Can you work these out from the model? Positions are in its coordinate system, mm. Face numbers are marked on the shaded views. Coordinates: 2 decimals unless noted, no trailing zeros. Loops run counter-clockwise (first coordinate to the right, second up) from the corner with the lowest first, then second, coordinate; pieces in that order, holes last. Notation, with made-up numbers: M 45,1.5 L 57,1.5 A18 cw 57,29.5 Z; hole C 83,-6 d7. An arc over 180 degrees is marked long. Answer as a JSON object with one key per item and string values. Group by question number.
Item 1: Suppose I cut it at A-A (x = 480). Write out the boundary of the cut face in (y, z).
Item 2: Suppose I cut it at D-D (y = -1327.5). Write out the boundary of the cut face in (x, z).
Item 3: Suppose I cut it at C-C (x = 410.5). Write out the boundary of the cut face in (y, z), then the cut area to 3 significant figures.
Item 4: Suppose I cut it at B-B (y = -1341.5). Write out the boundary of the cut face in (x, z), then the cut area to 3 significant figures.
Item 5: We'd pull the mould along X, two halves only. Please class the marked faces 1, 2, 3 and 4: +X half, -X half, draft (parallel to the pull), parting line (faces both ways), or undercut.
Item 6: If I drill on line 1 (X direction, y = -1322, z = 14.25); line 2 (X direction, y = -1331.5, z = 1.5); line 3 (Z direction, x = 560, y = -1330.5), over which ranges is the centre line in solid material (lowest first)?
Item 7: I'm going to push flat-ended pins straight in: pin 1 Ø3 at (x, y) = (397.81, -1294.47) entering from +Z; pin 2 Ø2.5 at (x, z) = (500.5, 2) entering from +Y; pin 3 Ø1.2 at (x, z) = (473, 16) entering from -Y. Where does each tip first touch, or does it pass through?
```python
from build123d import *

# Parameters (mm, degrees)
SKETCH1_W               = 214
SKETCH1_H               = 75.8
BOSS_EXTRUDE1_DEPTH     = 17
BOSSEXTENTION_DEPTH     = 214
SHELLIT_T               = -3
SKETCH7_W               = 208
SKETCH7_H               = 4
CUT_EXTRUDE4_DEPTH      = 3
SKETCH3_R               = 1.375
MOUNTING_HOLES_DEPTH    = 1479.493115905
PI_HOLE_DEPTH           = 8
CHAMFER1_START          = 8
CHAMFER1_DEPTH          = 2
CHAMFER1_START_2        = -970
CHAMFER1_2_DEPTH        = 1.564999152
FILLET1_R               = 2
SKETCH11_R              = 1.7
CUT_EXTRUDE5_DEPTH      = 893.868694268
CUT_EXTRUDE6_DEPTH      = 893.868694268
CUT_EXTRUDE6_DEPTH_BACK = 1
SKETCH12_R              = 2.75


with BuildPart() as part:
    # Sketch1 → Boss-Extrude1 (new body)
    with BuildSketch(Plane.XY):
        with Locations((466.705697041, -1324.673912477)):
            Rectangle(SKETCH1_W, SKETCH1_H)
    extrude(amount=BOSS_EXTRUDE1_DEPTH)

    # Sketch6 → BossExtention (add)
    with BuildSketch(Plane(origin=(573.705697041, 0, 0), x_dir=(0, 0, -1), z_dir=(1, 0, 0))):
        Polygon((-17, -1286.773912477), (-12.75, -1279.412696544), (0, -1286.773912477), align=None)
    extrude(amount=-BOSSEXTENTION_DEPTH)

    # Shellit
    shellit_openings = [part.faces().sort_by_distance(p)[0] for p in [
        (466.705697041, -1324.673912477, 17),
    ]]
    offset(amount=SHELLIT_T, openings=shellit_openings, kind=Kind.INTERSECTION)

    # Sketch7 → Cut-Extrude4 (cut)
    with BuildSketch(Plane.XY.offset(17)):
        with Locations((466.705697041, -1290.773912477)):
            Rectangle(SKETCH7_W, SKETCH7_H)
    extrude(amount=-CUT_EXTRUDE4_DEPTH, mode=Mode.SUBTRACT)

    # Sketch3 → Mounting Holes (cut, through all)
    with BuildSketch(Plane.XY.offset(3)):
        with Locations((397.805697041, -1294.473912477)):
            Circle(SKETCH3_R)
        with Locations((511.805697041, -1294.473912477)):
            Circle(SKETCH3_R)
        with Locations((397.805697041, -1353.573912477)):
            Circle(SKETCH3_R)
        with Locations((511.805697041, -1353.573912477)):
            Circle(SKETCH3_R)
    extrude(amount=-MOUNTING_HOLES_DEPTH, mode=Mode.SUBTRACT)

    # Sketch4 → PI_Hole (cut)
    with BuildSketch(Plane(origin=(0, 0, 0), x_dir=(-1, 0, 0), z_dir=(0, 0, -1))):
        with BuildLine():
            Line((-404.705697041, -1355.573912477), (-454.805697041, -1355.573912477))
            ThreePointArc((-454.805697041, -1355.573912477), (-456.219910604, -1356.159698914), (-456.805697041, -1357.573912477))
            Line((-456.805697041, -1357.573912477), (-456.805697041, -1358.073912477))
            ThreePointArc((-456.805697041, -1358.073912477), (-457.391483479, -1359.488126039), (-458.805697041, -1360.073912477))
            Line((-458.805697041, -1360.073912477), (-494.705697041, -1360.073912477))
            ThreePointArc((-494.705697041, -1360.073912477), (-496.119910604, -1359.488126039), (-496.705697041, -1358.073912477))
            Line((-496.705697041, -1358.073912477), (-496.705697041, -1357.573912477))
            ThreePointArc((-496.705697041, -1357.573912477), (-497.291483479, -1356.159698914), (-498.705697041, -1355.573912477))
            Line((-498.705697041, -1355.573912477), (-503.705697041, -1355.573912477))
            ThreePointArc((-503.705697041, -1355.573912477), (-505.827017385, -1354.69523282), (-506.705697041, -1352.573912477))
            Line((-506.705697041, -1352.573912477), (-506.705697041, -1338.573912477))
            ThreePointArc((-506.705697041, -1338.573912477), (-507.584376698, -1336.452592133), (-509.705697041, -1335.573912477))
            Line((-509.705697041, -1335.573912477), (-518.705697041, -1335.573912477))
            ThreePointArc((-518.705697041, -1335.573912477), (-520.827017385, -1334.69523282), (-521.705697041, -1332.573912477))
            Line((-521.705697041, -1332.573912477), (-521.705697041, -1311.773912477))
            ThreePointArc((-521.705697041, -1311.773912477), (-520.827017385, -1309.652592133), (-518.705697041, -1308.773912477))
            Line((-518.705697041, -1308.773912477), (-509.705697041, -1308.773912477))
            ThreePointArc((-509.705697041, -1308.773912477), (-507.584376698, -1307.89523282), (-506.705697041, -1305.773912477))
            Line((-506.705697041, -1305.773912477), (-506.705697041, -1295.773912477))
            ThreePointArc((-506.705697041, -1295.773912477), (-505.827017385, -1293.652592133), (-503.705697041, -1292.773912477))
            Line((-503.705697041, -1292.773912477), (-404.705697041, -1292.773912477))
            ThreePointArc((-404.705697041, -1292.773912477), (-402.584376698, -1293.652592133), (-401.705697041, -1295.773912477))
            Line((-401.705697041, -1295.773912477), (-401.705697041, -1352.573912477))
            ThreePointArc((-401.705697041, -1352.573912477), (-402.584376698, -1354.69523282), (-404.705697041, -1355.573912477))
        make_face()
    extrude(amount=-PI_HOLE_DEPTH, mode=Mode.SUBTRACT)

    # Chamfer1: read off the stored shape, not the designer's step
    # Chamfer1 outline → Chamfer1 (cut)
    with BuildSketch(Plane.XY.offset(CHAMFER1_START)):
        with BuildLine():
            ThreePointArc((457.482821386, -1359.573912477), (458.09859026, -1359.94474117), (458.805697041, -1360.073912477))
            Line((458.805697041, -1360.073912477), (494.705697041, -1360.073912477))
            ThreePointArc((494.705697041, -1360.073912477), (495.412803822, -1359.94474117), (496.028572697, -1359.573912477))
            Line((496.028572697, -1359.573912477), (457.482821386, -1359.573912477))
        make_face()
    extrude(amount=CHAMFER1_DEPTH, mode=Mode.SUBTRACT)

    # Chamfer1 2 outline → Chamfer1 2 (add)
    with BuildSketch(Plane(origin=(0, 0, 0), x_dir=(1, 0, 0), z_dir=(0, 0.70710678118655, -0.707106781186545)).offset(CHAMFER1_START_2)):
        with BuildLine():
            Line((494.705697041, 954.999972006), (458.805697041, 954.999972006))
            add(Edge.make_bspline(
                [(458.805697041, 954.999972006), (458.049768095, 954.999972006), (457.482821386, 954.292865225)],
                knots=[0, 0, 0, 0.722734248, 0.722734248, 0.722734248], degree=2, weights=[1, 0.935414347, 1]))
            Line((457.482821386, 954.292865225), (496.028572697, 954.292865225))
            add(Edge.make_bspline(
                [(496.028572697, 954.292865225), (495.461625987, 954.999972006), (494.705697041, 954.999972006)],
                knots=[5.560451059, 5.560451059, 5.560451059, 6.283185307, 6.283185307, 6.283185307], degree=2, weights=[1, 0.935414347, 1]))
        make_face()
    extrude(amount=CHAMFER1_2_DEPTH)

    # Fillet1
    fillet1_edges = [part.edges().sort_by_distance(p)[0] for p in [
        (359.705697041, -1324.673912477, 17),
        (573.705697041, -1283.09330451, 14.875),
        (359.705697041, -1283.09330451, 14.875),
        (466.705697041, -1362.573912477, 17),
        (573.705697041, -1324.673912477, 17),
        (573.705697041, -1362.573912477, 8.5),
        (359.705697041, -1362.573912477, 8.5),
        (466.705697041, -1286.773912477, 17),
    ]]
    fillet(fillet1_edges, radius=FILLET1_R)

    # Sketch11 → Cut-Extrude5 (cut, through all)
    with BuildSketch(Plane(origin=(0, -967.678510569, 558.689448566), x_dir=(1, 0, 0), z_dir=(0, -0.8660254037844403, 0.499999999999997))):
        with Locations(Location((466.705697041, -633.664524374, 0), (0, 0, 270))):
            Circle(SKETCH11_R)
        with Locations(Location((541.705697041, -633.664524374, 0), (0, 0, 270))):
            Circle(SKETCH11_R)
        with Locations(Location((391.705697041, -633.664524374, 0), (0, 0, 270))):
            Circle(SKETCH11_R)
    extrude(amount=-CUT_EXTRUDE5_DEPTH, mode=Mode.SUBTRACT)

    # Sketch12 → Cut-Extrude6 (cut, two sides: drawn at the far end of the back side and taken through both)
    with BuildSketch(Plane(origin=(0, -967.678510569, 558.689448566), x_dir=(1, 0, 0), z_dir=(0, -0.8660254037844403, 0.499999999999997)).offset(-CUT_EXTRUDE6_DEPTH_BACK)):
        with Locations(Location((391.705697041, -633.664524374, 0), (0, 0, 46.658241773))):
            Circle(SKETCH12_R)
        with Locations(Location((466.705697041, -633.664524374, 0), (0, 0, 46.658241773))):
            Circle(SKETCH12_R)
        with Locations(Location((541.705697041, -633.664524374, 0), (0, 0, 46.658241773))):
            Circle(SKETCH12_R)
    extrude(amount=CUT_EXTRUDE6_DEPTH + CUT_EXTRUDE6_DEPTH_BACK, mode=Mode.SUBTRACT)


solid = part.part
```
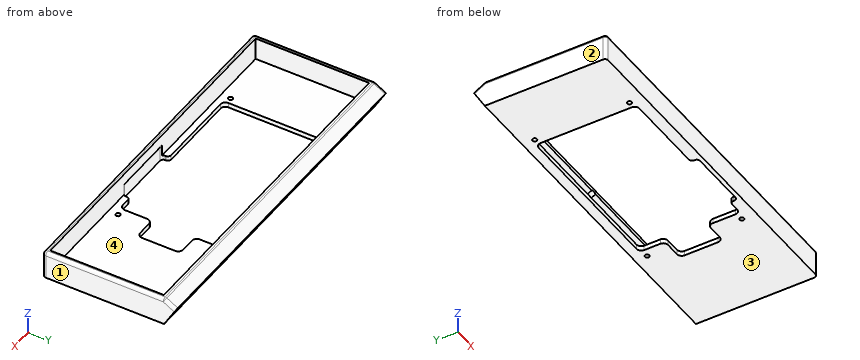
From the geometry:
{
 "1": {"outline": "M -1362.57,0 L -1360.07,0 L -1360.07,9.5 L -1359.57,10 L -1359.57,17 L -1360.57,17 A2 ccw -1362.57,15 Z; M -1292.77,0 L -1286.77,0 L -1279.41,12.75 L -1286.31,16.73 A2 ccw -1287.31,17 L -1288.77,17 L -1288.77,14.69 L -1283.51,11.65 L -1288.51,3 L -1292.77,3 Z"},
 "2": {"outline": "M 359.71,0 L 401.71,0 L 401.71,3 L 362.71,3 L 362.71,17 L 361.71,17 A2 ccw 359.71,15 Z; M 521.71,0 L 573.71,0 L 573.71,15 A2 ccw 571.71,17 L 570.71,17 L 570.71,3 L 521.71,3 Z"},
 "3": {"outline": "M -1362.57,0 L -1355.57,0 L -1355.57,3 L -1359.57,3 L -1359.57,17 L -1360.57,17 A2 ccw -1362.57,15 Z; M -1292.77,0 L -1286.77,0 L -1279.41,12.75 L -1286.31,16.73 A2 ccw -1287.31,17 L -1288.77,17 L -1288.77,14.69 L -1283.51,11.65 L -1288.51,3 L -1292.77,3 Z", "area": "139 mm2"},
 "4": {"outline": "M 359.71,0 L 401.71,0 L 401.71,3 L 362.71,3 L 362.71,17 L 361.71,17 A2 ccw 359.71,15 Z; M 506.71,0 L 573.71,0 L 573.71,15 A2 ccw 571.71,17 L 570.71,17 L 570.71,3 L 506.71,3 Z", "area": "409 mm2"},
 "5": {"face 1": "+X half", "face 2": "-X half", "face 3": "draft", "face 4": "undercut"},
 "6": {"line 1": "359.71 to 362.71, 570.71 to 573.71", "line 2": "359.71 to 401.71, 521.71 to 573.71", "line 3": "0 to 3"},
 "7": {"pin 1": "z = 3", "pin 2": "y = -1284.9", "pin 3": "y = -1362.53"}
}
